from build123d import *

# Parameters (mm, degrees)
EXTRUDE_1_DEPTH     = 12
SKETCH_1_3_R        = 3.63567385
CUT_EXTRUDE_1_DEPTH = 12
SKETCH_2_R          = 7.5
CUT_EXTRUDE_2_DEPTH = 5
SKETCH_4_R          = 12.5
EXTRUDE_2_DEPTH     = 12
SKETCH_5_W          = 40
SKETCH_5_H          = 88
EXTRUDE_3_DEPTH     = 4
FILLET_1_R          = 16


with BuildPart() as part:
    # Sketch 1 → Extrude 1 (new body)
    with BuildSketch(Plane(origin=(0, 0, 0), x_dir=(1, 0, 0), z_dir=(0, 1, 0))):
        with BuildLine():
            Line((-50, 36), (50, 36))
            Line((50, 36), (50, -20))
            ThreePointArc((50, -20), (45.313708499, -31.313708499), (34, -36))
            Line((34, -36), (-34, -36))
            ThreePointArc((-34, -36), (-45.313708499, -31.313708499), (-50, -20))
            Line((-50, -20), (-50, 36))
        make_face()
    extrude(amount=EXTRUDE_1_DEPTH)

    # Sketch 1_3 → Cut-Extrude 1 (cut)
    with BuildSketch(Plane(origin=(0, 0, 0), x_dir=(1, 0, 0), z_dir=(0, 1, 0))):
        with Locations(Location((34, -20, 0), (0, 0, 270))):
            Circle(SKETCH_1_3_R)
        with Locations(Location((-34, -20, 0), (0, 0, 270))):
            Circle(SKETCH_1_3_R)
    extrude(amount=CUT_EXTRUDE_1_DEPTH, mode=Mode.SUBTRACT)

    # Sketch 2 → Cut-Extrude 2 (cut)
    with BuildSketch(Plane(origin=(0, 12, 0), x_dir=(1, 0, 0), z_dir=(0, 1, 0))):
        with Locations(Location((34, -20, 0), (0, 0, 270))):
            Circle(SKETCH_2_R)
        with Locations(Location((-34, -20, 0), (0, 0, 270))):
            Circle(SKETCH_2_R)
    extrude(amount=-CUT_EXTRUDE_2_DEPTH, mode=Mode.SUBTRACT)

    # Sketch 4 → Extrude 2 (add)
    with BuildSketch(Plane(origin=(0, 0, -36), x_dir=(-1, 0, 0), z_dir=(0, 0, -1))):
        with BuildLine():
            Line((-30, 12), (30, 12))
            Line((30, 12), (30, 120))
            ThreePointArc((30, 120), (0, 150), (-30, 120))
            Line((-30, 120), (-30, 12))
        make_face()
        with Locations((0, 120)):
            Circle(SKETCH_4_R, mode=Mode.SUBTRACT)
    extrude(amount=-EXTRUDE_2_DEPTH)

    # Sketch 5 → Extrude 3 (add, symmetric)
    with BuildSketch(Plane(origin=(0, 0, 0), x_dir=(0, 0, -1), z_dir=(1, 0, 0))):
        with Locations((4, 56)):
            Rectangle(SKETCH_5_W, SKETCH_5_H)
    extrude(amount=EXTRUDE_3_DEPTH, both=True)

    # Fillet 1
    fillet_1_edges = [part.edges().sort_by_distance(p)[0] for p in [
        (0, 100, 16),
    ]]
    fillet(fillet_1_edges, radius=FILLET_1_R)


solid = part.part
Verification items for the finished model (mm, model axes). A direction names the side the tool comes from. Give positions to 0.01 mm unless a question says otherwise; leave off trailing zeros. Order: outer loops, then holes, each group sorted by start corner. A loop starts at its lowest first (then second) coordinate and runs counter-clockwise, first axis right, second up. Notation, with made-up numbers: M 88.5,88 L 121.5,88 A12 ccw 121.5,108 Z; hole C 83.5,77 d5. An arc over 180 degrees is marked long. Use one line per item in the form item = value. Start each with the question number.
Q1. Scan lines: line 1 along X through (y, z) = (2, 20); line 2 along X through (y, z) = (10, 20); line 3 along Z through (x, y) = (34, 5.75). Record each from-to range of solid material in increasing order. Write a range as [from, to].
Q2. Section check C-C (y = 54). Enter the section's corners in (x, z).
Q3. Section check B-B (y = 9). Enter the section's corners in (x, z), then the cut area to 3 significant figures.
Q4. Access from +Z, -Z, +X, -X, +Y, -Y to the whole of each face (thin tool, end or side, straight path). Record for faces 1 (the cylindrical face through (1.627, 132.394, -30.084)), 2 (the flat face through (0, 47, 16)), 3 (the cylindrical face through (-38.564, 9.535, 14.048)), 4 (the flat face through (-4, 57, -4)).
Q5. Section check A-A (x = 0). Enter the section's corners in (y, z), then the cut area to 3 significant figures.
Q6. Mould release check, pull along Z, two halves, no side actions. Record for faces 5 (the cylindrical face through (-37.225, 3.451, 21.678)), 6 (the cylindrical face through (-0.056, 95.189, 11.437)), 7 (the flat face through (30, 67, -30)): +Z half, -Z half, draft (parallel to the pull), parting line (faces both ways), or undercut.
Q7. Section check D-D (z = -13.5). Enter the section's corners in (x, y).
Q8. Go/stop test with flat-tipped pins: pin 1 Ø4.5 at (x, z) = (35, 16.5) entering from +Y; pin 2 Ø6.5 at (x, z) = (-1, -17) entering from +Y; pin 3 Ø3.5 at (y, z) = (91, -29.5) entering from -X; pin 4 Ø1.5 at (x, z) = (16, 18.5) entering from -Y. Record where each tip stops, or that it passes through.
Evaluation:
q1.line_1 = [-50, -37.64], [-30.36, 30.36], [37.64, 50]
q1.line_2 = [-50, -41.5], [-26.5, 26.5], [41.5, 50]
q1.line_3 = [-36, 16.36], [23.64, 36]
q2.outline = M -30,-36 L 30,-36 L 30,-24 L 4,-24 L 4,16 L -4,16 L -4,-24 L -30,-24 Z
q3.outline = M -50,-36 L 50,-36 L 50,20 A16 ccw 34,36 L -34,36 A16 ccw -50,20 Z; hole C -34,20 d15; hole C 34,20 d15
q3.area = 6,740 mm2
q4.face_1 = +Z, -Z
q4.face_2 = +Z, +X, -X, +Y
q4.face_3 = +Y
q4.face_4 = +Z, -X, +Y
q5.outline = M 0,-36 L 107.5,-36 L 107.5,-24 L 100,-24 L 100,0 A16 ccw 84,16 L 12,16 L 12,36 L 0,36 Z; M 132.5,-36 L 150,-36 L 150,-24 L 132.5,-24 Z
q5.area = 5,690 mm2
q6.face_5 = undercut
q6.face_6 = +Z half
q6.face_7 = draft
q7.outline = M -50,0 L 50,0 L 50,12 L 4,12 L 4,100 L -4,100 L -4,12 L -50,12 Z
q8.pin_1 = 7
q8.pin_2 = 100
q8.pin_3 = -30
q8.pin_4 = 0
